```python
from build123d import *

# Parameters (mm, degrees)
F0_R     = 19.05
F1_DEPTH = 15.875
F2_R     = 9.525
F3_DEPTH = 12.7
F4_R     = 1.5875
F5_DEPTH = 50.8
F6_R     = 1.5875
F7_DEPTH = 50.8


with BuildPart() as f1:
    # F0 (on Front) → F1 (new body)
    with BuildSketch(Plane.XZ):
        Circle(F0_R)
    extrude(amount=F1_DEPTH)

    # F2 (on face) → F3 (join)
    with BuildSketch(Plane.XZ.offset(15.875)):
        Circle(F2_R)
    extrude(amount=F3_DEPTH)

    # F4 (on face) → F5 (cut)
    with BuildSketch(Plane.XZ.offset(28.575)):
        with Locations((0, 7.356282)):
            Circle(F4_R)
    extrude(amount=-F5_DEPTH, mode=Mode.SUBTRACT)

    # F6 (on face) → F7 (cut)
    with BuildSketch(Plane.XZ.offset(28.575)):
        with Locations((-4.208875, 5.569106)):
            Circle(F6_R)
    extrude(amount=-F7_DEPTH, mode=Mode.SUBTRACT)


solid = f1.part
```
The model under review builds one solid part; all positions refer to its coordinate system, in mm. Give positions to 0.01 mm unless a question says otherwise; leave off trailing zeros. Write each loop counter-clockwise with the first axis right and the second up, starting at its lowest first coordinate (ties: lowest second). Pieces come first, ordered by that corner, then holes.
(1) Consider section D-D, the plane x = 8. Give the boundary of the cut face in (y, z) (3 decimals), and give its area (3 significant figures).
(2) Consider section B-B, the plane z = 0. Give the boundary of the cut face in (x, y) (3 decimals), and give its area (3 significant figures).
(3) Consider section A-A, the plane x = 0. Give the boundary of the cut face in (y, z) (3 decimals).
(4) The part is to be moulded in two halves that separate along X. For faces 1 (the cylindrical face through (-0.344, -14.488, 5.807)), 2 (the cylindrical face through (-7.559, -22.136, -5.796)), 3 (the flat face through (4, -15.875, 9)), say which applies: released by +X, released by -X, zero draft, split by the parting line, or undercut.
(5) To check wall thickness, follow L1, parallel to Z at x = 0, y = -11.25; L2, parallel to Z at x = 0, y = -17.5 (3 decimals); L3, parallel to Y at x = 7.5, z = -10.5 (3 decimals). State the ranges of each line that lie inside material, in increasing order.
(6) Consider section C-C, the plane y = -18.75. Give the number of separate pieces and of enclosed holes in the cut face, and give its area (3 significant figures).
(7) For P1, Ø8, axis at x = -7, y = -5.5, coming from the -Z side; P2, Ø1, axis at x = -7, z = -13, coming from the -Y side (3 decimals); P3, Ø6, axis at x = 7.5, y = -10.5, coming from the +Z side, all flat-tipped, find the tip position at first contact; note any pin that passes through.
Returned:
1. outline: (-28.575, -5.17) - (-15.875, -5.17) - (-15.875, -17.289) - (0, -17.289) - (0, 17.289) - (-15.875, 17.289) - (-15.875, 5.17) - (-28.575, 5.17) - close
1. area: 680 mm2
2. outline: (-19.05, -15.875) - (-9.525, -15.875) - (-9.525, -28.575) - (9.525, -28.575) - (9.525, -15.875) - (19.05, -15.875) - (19.05, 0) - (-19.05, 0) - close
2. area: 847 mm2
3. outline: (-28.575, -9.525) - (-15.875, -9.525) - (-15.875, -19.05) - (0, -19.05) - (0, 5.769) - (-28.575, 5.769) - close; (-28.575, 8.944) - (0, 8.944) - (0, 19.05) - (-15.875, 19.05) - (-15.875, 9.525) - (-28.575, 9.525) - close
4. face 1: undercut
4. face 2: split by the parting line
4. face 3: zero draft
5. L1: z = -19.05 to 5.77, 8.94 to 19.05
5. L2: z = -9.525 to 5.769, 8.944 to 9.525
5. L3: y = -15.875 to 0
6. separate pieces: 1
6. enclosed holes: 2
6. area: 269 mm2
7. P1: stops at z = -18.81
7. P2: stops at y = -15.875
7. P3: stops at z = 18.51
